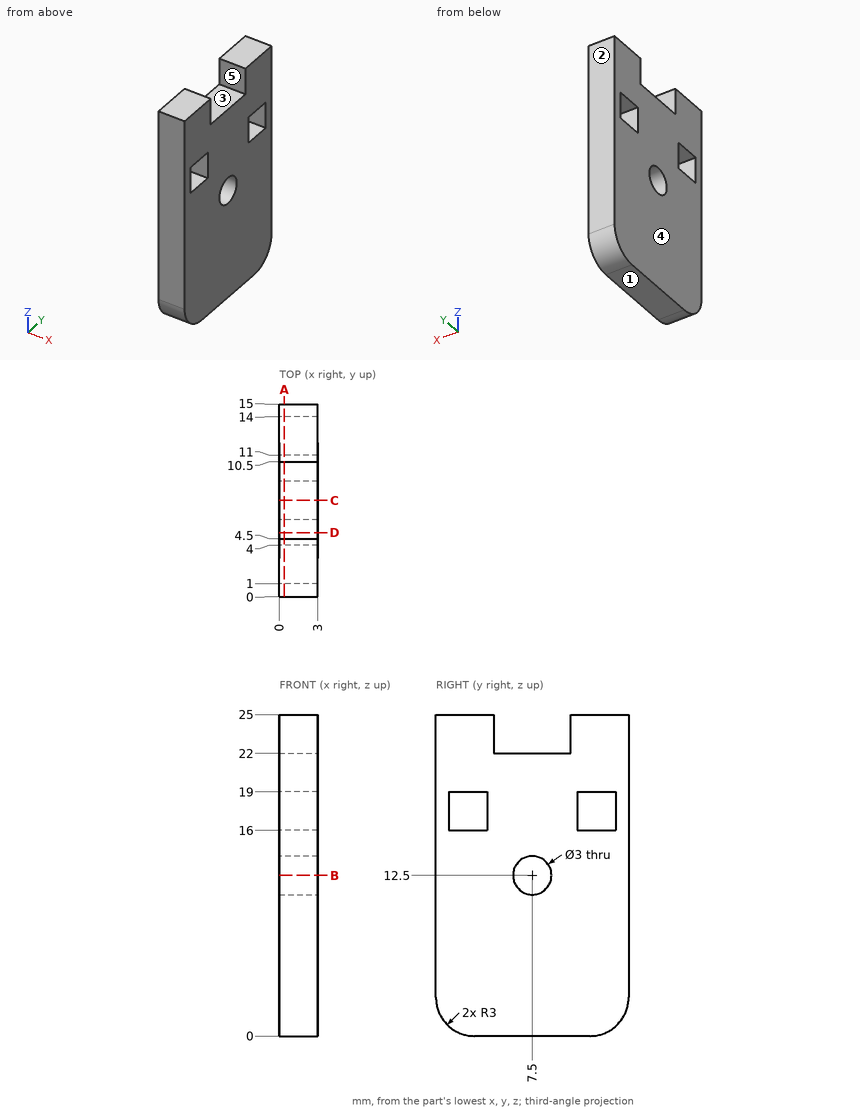
Study the drawing (mm; zero at the part's minimum x, y, z) and answer. A direction names the side the tool comes from. Give positions to 0.01 mm unless a question says otherwise; leave off trailing zeros. Write each loop counter-clockwise with the first axis right and the second up, starting at its lowest first coordinate (ties: lowest second). Pieces come first, ordered by that corner, then holes.
(1) The part is cut by section D-D on y = 5. Write down the section's boundary in (x, z).
Final values:
outline: (0, 0) - (3, 0) - (3, 22) - (0, 22) - close
(2) A flat-ended cylindrical pin translates along its axis: pin 1 Ø0.9 at (x, y) = (2, 6.5) entering from +Z. Find the tip coordinate at first contact, or state that the pin passes through.
Final values:
pin 1: stops at z = 22
(3) The part is cut by section A-A on x = 0.4. Write down the section's boundary in (y, z).
Final values:
outline: (0, 3) arc R3 ccw to (3, 0) - (12, 0) arc R3 ccw to (15, 3) - (15, 25) - (10.5, 25) - (10.5, 22) - (4.5, 22) - (4.5, 25) - (0, 25) - close; hole (1, 16) - (4, 16) - (4, 19) - (1, 19) - close; hole circle Ø3 at (7.5, 12.5); hole (11, 16) - (14, 16) - (14, 19) - (11, 19) - close
(4) The part is cut by section B-B on z = 12.5. Write down the section's boundary in (x, y).
Final values:
outline: (0, 0) - (3, 0) - (3, 6) - (0, 6) - close; (0, 9) - (3, 9) - (3, 15) - (0, 15) - close
(5) Straight lines are drawn through the part: line 1 (Y direction, x = 1.8, z = 12.5); line 2 (Z direction, x = 1.5, y = 11.5); line 3 (Y direction, x = 1.8, z = 23.5). For each, find the intervals that lie inside material, in ascending order.
Final values:
line 1: y = 0 to 6, 9 to 15
line 2: z = 0 to 16, 19 to 25
line 3: y = 0 to 4.5, 10.5 to 15
(6) Which of the six approach directions +Z, -Z, +X, -X, +Y, -Y give full straight-line access (tool end or side, diameter ignored) to the marked faces 4 and 5?
Final values:
face 4: +Z, -Z, -X, +Y, -Y
face 5: +Z, +X, -X
(7) The part is cut by section C-C on y = 7.5. Write down the section's boundary in (x, z), plus the area to 3 significant figures.
Final values:
outline: (0, 0) - (3, 0) - (3, 11) - (0, 11) - close; (0, 14) - (3, 14) - (3, 22) - (0, 22) - close
area: 57.0 mm2
(8) The mould has two halves that part along Y. Classify the marked faces 1, 2 and 3: pulls with the +Y half, pulls with the -Y half, needs draft (parallel to the pull), parting line crosses it, or undercut.
Final values:
face 1: needs draft
face 2: pulls with the +Y half
face 3: undercut
